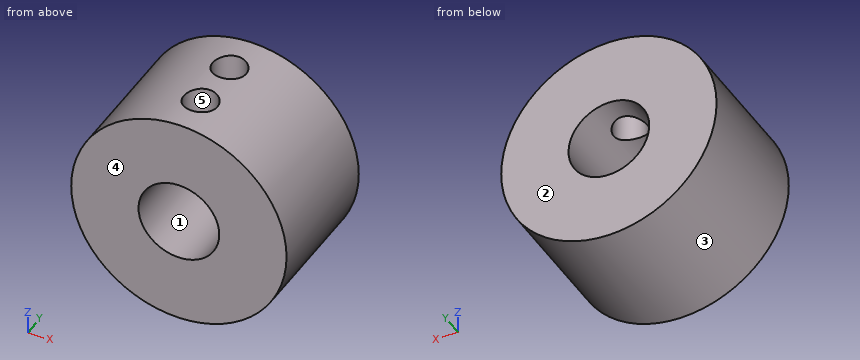
```python
from build123d import *

# Parameters (mm, degrees)
SKETCH1_R           = 12.7
BOSS_EXTRUDE1_DEPTH = 15.875
SKETCH2_R           = 4.7625
CUT_EXTRUDE1_DEPTH  = 24.970724332
SKETCH3_R           = 1.984375
CUT_EXTRUDE2_DEPTH  = 24.970724332


with BuildPart() as part:
    # Sketch1 → Boss-Extrude1 (new body)
    with BuildSketch(Plane(origin=(0, 0, 0), x_dir=(1, 0, 0), z_dir=(0, 1, 0))):
        with Locations(Location((0, 0, 0), (0, 0, 270))):
            Circle(SKETCH1_R)
    extrude(amount=BOSS_EXTRUDE1_DEPTH)

    # Sketch2 → Cut-Extrude1 (cut, through all)
    with BuildSketch(Plane(origin=(0, 15.875, 0), x_dir=(1, 0, 0), z_dir=(0, 1, 0))):
        with Locations(Location((0, 0, 0), (0, 0, 270))):
            Circle(SKETCH2_R)
    extrude(amount=-CUT_EXTRUDE1_DEPTH, mode=Mode.SUBTRACT)

    # Sketch3 → Cut-Extrude2 (cut, through all)
    with BuildSketch(Plane.XY):
        with Locations(Location((0, 4.7625, 0), (0, 0, 90.000000002))):
            Circle(SKETCH3_R)
        with Locations(Location((0, 11.1125, 0), (0, 0, 90.000000002))):
            Circle(SKETCH3_R)
    extrude(amount=CUT_EXTRUDE2_DEPTH, mode=Mode.SUBTRACT)


solid = part.part
```
Input: part model. Units: mm. Frame: model coordinates. Face numbers are marked on the shaded views. A direction names the side the tool comes from. Coordinates: 2 decimals unless noted, no trailing zeros. Loops run counter-clockwise (first coordinate to the right, second up) from the corner with the lowest first, then second, coordinate; pieces in that order, holes last.
Q1. Line query: line 1 along Y through (x, z) = (0, 6.5) (3 decimals); line 2 along X through (y, z) = (6, 0); line 3 along Z through (x, y) = (2.25, 11.25). Output: solid intervals per line, ascending.
Results are:
line 1: y = 0 to 2.778, 6.747 to 9.128, 13.097 to 15.875
line 2: x = -12.7 to -4.76, 4.76 to 12.7
line 3: z = -12.5 to -4.2, 4.2 to 12.5
Q2. Section C-C, the plane x = 8.5. Return the cut outline in (y, z) (3 decimals).
Results are:
outline: (0, -9.436) - (15.875, -9.436) - (15.875, 9.436) - (0, 9.436) - close
Q3. Section D-D, the plane y = 4. Return the cut outline in (x, z) (1 decimal), and give its area (3 significant figures).
Results are:
outline: (-1.8, 4.4) - (-1.8, 12.6) arc R12.7 ccw (long way) to (1.8, 12.6) - (1.8, 4.4) arc R4.8 cw (long way) to start
area: 406 mm2
Q4. Section B-B, the plane z = 0. Return the cut outline in (x, y) (1 decimal).
Results are:
outline: (-12.7, 0) - (-4.8, 0) - (-4.8, 15.9) - (-12.7, 15.9) - close; (4.8, 0) - (12.7, 0) - (12.7, 15.9) - (4.8, 15.9) - close
Q5. Contact query for flat-ended pins moving along their axis: pin 1 (1.5 mm diameter, centred on x = 9, y = 13.5, fed in from -Z); pin 2 (3 mm diameter, centred on x = -9, y = 3, fed in from +Z); pin 3 (6 mm diameter, centred on x = -6.5, y = 9, fed in from -Z). Output: stop coordinate, or through.
Results are:
pin 1: stops at z = -9.66
pin 2: stops at z = 10.25
pin 3: stops at z = -12.21
Q6. Set-up query: the marked faces 4 and 5. Return all of +Z, -Z, +X, -X, +Y, -Y with unobstructed straight access to the full face (end or side cutting, diameter ignored); none if empty.
Results are:
face 4: +Z, -Z, +X, -X, -Y
face 5: +Z
Q7. Mould query, pull axis X, two halves, no side actions, for the marked faces 1, 2 and 3. Classes: +X half, -X half, draft (parallel to the pull), parting line (faces both ways), or undercut.
Results are:
face 1: undercut
face 2: draft
face 3: parting line
Q8. Section A-A, the plane x = 0. Return the cut outline in (y, z) (1 decimal), and give its area (3 significant figures).
Results are:
outline: (0, -12.7) - (15.9, -12.7) - (15.9, -4.8) - (0, -4.8) - close; (0, 4.8) - (2.8, 4.8) - (2.8, 12.7) - (0, 12.7) - close; (6.7, 4.8) - (9.1, 4.8) - (9.1, 12.7) - (6.7, 12.7) - close; (13.1, 4.8) - (15.9, 4.8) - (15.9, 12.7) - (13.1, 12.7) - close
area: 189 mm2
